from build123d import *

# Parameters (mm, degrees)
BOSS_EXTRUDE1_DEPTH      = 5
SKETCH2_W                = 1
SKETCH2_H                = 2
SKETCH2_W_2              = 2
SKETCH2_H_2              = 30.5
BOSS_EXTRUDE2_DEPTH      = 2
FILLET1_R                = 4
BOSS_EXTRUDE3_DEPTH      = 5
BOSS_EXTRUDE3_DEPTH_BACK = 0.5
SKETCH3_R                = 0.75
FILLET3_R                = 1


with BuildPart() as part:
    # Sketch1 → Boss-Extrude1 (new body)
    with BuildSketch(Plane(origin=(0, 0, 0), x_dir=(1, 0, 0), z_dir=(0, 1, 0))):
        with BuildLine():
            Line((0, 14.4), (25, 14.4))
            ThreePointArc((25, 14.4), (39.4, 0), (25, -14.4))
            Line((25, -14.4), (0, -14.4))
            ThreePointArc((0, -14.4), (-14.4, 0), (0, 14.4))
        make_face()
        with BuildLine():
            Line((0, 12.4), (25, 12.4))
            ThreePointArc((25, 12.4), (37.4, 0), (25, -12.4))
            Line((25, -12.4), (0, -12.4))
            ThreePointArc((0, -12.4), (-12.4, 0), (0, 12.4))
        make_face(mode=Mode.SUBTRACT)
    extrude(amount=BOSS_EXTRUDE1_DEPTH)

    # Sketch2 → Boss-Extrude2 (add)
    with BuildSketch(Plane.XZ):
        with Locations((56.9, 32.5)):
            Rectangle(SKETCH2_W, SKETCH2_H)
        with Locations((55.4, 32.5)):
            Rectangle(SKETCH2_W_2, SKETCH2_H)
        with Locations((55.4, 16.25)):
            Rectangle(SKETCH2_W_2, SKETCH2_H_2)
        with BuildLine():
            Line((39.365235814, -1), (54.4, -1))
            Line((54.4, -1), (54.4, 1))
            Line((54.4, 1), (39.365235814, 1))
            ThreePointArc((39.365235814, 1), (39.4, 0), (39.365235814, -1))
        make_face()
        with Locations((55.4, 0)):
            Rectangle(SKETCH2_W_2, SKETCH2_H)
        with BuildLine():
            Line((37.4, -1), (39.365235814, -1))
            ThreePointArc((39.365235814, -1), (39.4, 0), (39.365235814, 1))
            Line((39.365235814, 1), (37.4, 1))
            Line((37.4, 1), (37.4, -1))
        make_face()
    extrude(amount=-BOSS_EXTRUDE2_DEPTH)

    # Fillet1
    # the kernel refuses this fillet: 4 mm, written as the material it adds along each edge
    with BuildSketch(Plane(origin=(25, 2, 0), x_dir=(0.7371891614816782, 0, -0.6756864214959037), z_dir=(-0.6756864214959037, 0, -0.7371891614816782))) as fillet1_piece_1_section:
        with BuildLine():
            CenterArc((18.272983346, -4), FILLET1_R, 90, 75.522487814)
            Line((18.272983346, 0), (18.272983346, 0.08))
            Line((18.272983346, 0.08), (14.4, 0.08))
            Line((14.4, 0.08), (14.32, 0))
            ThreePointArc((14.32, 0), (14.32, -1.5), (14.322540333, -2.98))
            Line((14.322540333, -2.98), (14.4, -3))
        make_face()
    fillet1_piece_1 = revolve(axis=Axis((25, 2, 0), (0, -1, 0)), revolution_arc=85.014954966, mode=Mode.PRIVATE)
    fillet1_piece_1 = split(fillet1_piece_1, bisect_by=Plane(origin=(40.301586348, 2.758397987, -1), z_dir=(0, 0, 1)), keep=Keep.TOP, mode=Mode.PRIVATE)
    fillet1_piece_1 = split(fillet1_piece_1, bisect_by=Plane(origin=(40.301586348, 2.758397987, 1), z_dir=(0, 0, -1)), keep=Keep.TOP, mode=Mode.PRIVATE)
    add(fillet1_piece_1)
    with BuildSketch(Plane(origin=(39.365235814, 2, 1), x_dir=(-0.17149804582148107, 0, 0.9851844600273663), z_dir=(0, -1, 0))) as fillet1_piece_2:
        with BuildLine():
            CenterArc((3.367524545, -3.978862537), FILLET1_R, 95.892851455, 74.232218513)
            Line((-0.573213295, -3.292870354), (-0.652028052, -3.27915051))
            Line((-0.652028052, -3.27915051), (-0.078814757, 0.013719844))
            Line((-0.078814757, 0.013719844), (0.008213474, 0.079577251))
            ThreePointArc((0.008213474, 0.079577251), (1.47842541, 0.003905135), (2.948637345, 0.079577251))
            Line((2.948637345, 0.079577251), (2.95685082, 0))
        make_face()
    extrude(amount=2)
    with BuildSketch(Plane(origin=(39.365235814, 2, -1), x_dir=(-0.17149804582148342, 0, -0.9851844600273658), z_dir=(0, -1, 0))) as fillet1_piece_3:
        with BuildLine():
            CenterArc((3.367524545, 3.978862537), FILLET1_R, 189.874930032, 74.232218513)
            Line((-0.573213295, 3.292870354), (-0.652028052, 3.27915051))
            Line((-0.652028052, 3.27915051), (-0.078814757, -0.013719844))
            Line((-0.078814757, -0.013719844), (0.008213474, -0.079577251))
            ThreePointArc((0.008213474, -0.079577251), (1.47842541, -0.003905135), (2.948637345, -0.079577251))
            Line((2.948637345, -0.079577251), (2.95685082, 0))
        make_face()
    extrude(amount=2)
    with BuildSketch(Plane(origin=(54.4, 0, 1), x_dir=(-1, 0, 0), z_dir=(0, 1, 0))) as fillet1_piece_4:
        with BuildLine():
            CenterArc((FILLET1_R, FILLET1_R), FILLET1_R, 180, 90)
            Line((0, FILLET1_R), (-FILLET1_R * 0.02, FILLET1_R))
            Line((-FILLET1_R * 0.02, FILLET1_R), (-FILLET1_R * 0.02, -FILLET1_R * 0.02))
            Line((-FILLET1_R * 0.02, -FILLET1_R * 0.02), (FILLET1_R, -FILLET1_R * 0.02))
            Line((FILLET1_R, -FILLET1_R * 0.02), (FILLET1_R, 0))
        make_face()
    extrude(amount=2)
    with BuildSketch(Plane(origin=(56.4, 0, 31.5), x_dir=(0, 0, -1), z_dir=(0, 1, 0))) as fillet1_piece_5:
        with BuildLine():
            CenterArc((2.645751311, -4), FILLET1_R, 90, 41.409622109)
            Line((0, -1), (-0.052915026, -0.94))
            ThreePointArc((-0.052915026, -0.94), (-0.08, -0.5), (-0.08, 0))
            Line((-0.08, 0), (0, 0.08))
            Line((0, 0.08), (2.645751311, 0.08))
            Line((2.645751311, 0.08), (2.645751311, 0))
        make_face()
    extrude(amount=2)
    with BuildSketch(Plane(origin=(39.365235814, 10.355974154, -1), x_dir=(-0.1714980458214834, 0, -0.9851844600273658), z_dir=(0, -1, 0))) as fillet1_piece_6a_section:
        with BuildLine():
            CenterArc((3.367524545, 3.978862537), FILLET1_R, 189.874930032, 74.232218513)
            Line((-0.573213295, 3.292870354), (-0.652028052, 3.27915051))
            Line((-0.652028052, 3.27915051), (-0.078814757, -0.013719844))
            Line((-0.078814757, -0.013719844), (0.008213474, -0.079577251))
            ThreePointArc((0.008213474, -0.079577251), (1.47842541, -0.003905135), (2.948637345, -0.079577251))
            Line((2.948637345, -0.079577251), (2.95685082, 0))
        make_face()
    fillet1_piece_6a = extrude(amount=10.355974154, mode=Mode.PRIVATE)
    fillet1_piece_6a = split(fillet1_piece_6a, bisect_by=Plane(origin=(40.057221624, 5, -1.646357347), z_dir=(0, -1, 0)), keep=Keep.TOP, mode=Mode.PRIVATE)
    fillet1_piece_6a = split(fillet1_piece_6a, bisect_by=Plane(origin=(40.057221624, 2, -1.646357347), z_dir=(0, 1, 0)), keep=Keep.TOP, mode=Mode.PRIVATE)
    with BuildSketch(Plane(origin=(25, 2, 0), x_dir=(0.7371891614816782, 0, -0.6756864214959037), z_dir=(-0.6756864214959037, 0, -0.7371891614816782))) as fillet1_piece_6b_section:
        with BuildLine():
            CenterArc((18.272983346, -4), FILLET1_R, 90, 75.522487814)
            Line((18.272983346, 0), (18.272983346, 0.08))
            Line((18.272983346, 0.08), (14.4, 0.08))
            Line((14.4, 0.08), (14.32, 0))
            ThreePointArc((14.32, 0), (14.32, -1.5), (14.322540333, -2.98))
            Line((14.322540333, -2.98), (14.4, -3))
        make_face()
    fillet1_piece_6b = revolve(axis=Axis((25, 2, 0), (0, -1, 0)), revolution_arc=85.014954966, mode=Mode.PRIVATE)
    fillet1_piece_6b = split(fillet1_piece_6b, bisect_by=Plane(origin=(38.861424428, 2.733448244, -1), z_dir=(0, 0, -1)), keep=Keep.TOP, mode=Mode.PRIVATE)
    fillet1_piece_6 = fillet1_piece_6a & fillet1_piece_6b
    add(fillet1_piece_6)
    with BuildSketch(Plane(origin=(25, 2, 0), x_dir=(0.7371891614816782, 0, -0.6756864214959037), z_dir=(-0.6756864214959037, 0, -0.7371891614816782))) as fillet1_piece_7a_section:
        with BuildLine():
            CenterArc((18.272983346, -4), FILLET1_R, 90, 75.522487814)
            Line((18.272983346, 0), (18.272983346, 0.08))
            Line((18.272983346, 0.08), (14.4, 0.08))
            Line((14.4, 0.08), (14.32, 0))
            ThreePointArc((14.32, 0), (14.32, -1.5), (14.322540333, -2.98))
            Line((14.322540333, -2.98), (14.4, -3))
        make_face()
    fillet1_piece_7a = revolve(axis=Axis((25, 2, 0), (0, -1, 0)), revolution_arc=85.014954966, mode=Mode.PRIVATE)
    fillet1_piece_7a = split(fillet1_piece_7a, bisect_by=Plane(origin=(38.861423807, 2.733448455, 1), z_dir=(0, 0, 1)), keep=Keep.TOP, mode=Mode.PRIVATE)
    with BuildSketch(Plane(origin=(39.365235814, 10.355974154, 1), x_dir=(-0.17149804582148107, 0, 0.9851844600273663), z_dir=(0, -1, 0))) as fillet1_piece_7b_section:
        with BuildLine():
            CenterArc((3.367524545, -3.978862537), FILLET1_R, 95.892851455, 74.232218513)
            Line((-0.573213295, -3.292870354), (-0.652028052, -3.27915051))
            Line((-0.652028052, -3.27915051), (-0.078814757, 0.013719844))
            Line((-0.078814757, 0.013719844), (0.008213474, 0.079577251))
            ThreePointArc((0.008213474, 0.079577251), (1.47842541, 0.003905135), (2.948637345, 0.079577251))
            Line((2.948637345, 0.079577251), (2.95685082, 0))
        make_face()
    fillet1_piece_7b = extrude(amount=10.355974154, mode=Mode.PRIVATE)
    fillet1_piece_7b = split(fillet1_piece_7b, bisect_by=Plane(origin=(40.057221624, 5, 1.646357347), z_dir=(0, -1, 0)), keep=Keep.TOP, mode=Mode.PRIVATE)
    fillet1_piece_7b = split(fillet1_piece_7b, bisect_by=Plane(origin=(40.057221624, 2, 1.646357347), z_dir=(0, 1, 0)), keep=Keep.TOP, mode=Mode.PRIVATE)
    fillet1_piece_7 = fillet1_piece_7a & fillet1_piece_7b
    add(fillet1_piece_7)
    # the kernel refuses this fillet: 4 mm, written as the material it takes off along each edge
    with BuildSketch(Plane(origin=(56.4, -10, -1), x_dir=(-1, 0, 0), z_dir=(0, 1, 0))) as fillet1_2_piece_1:
        with BuildLine():
            CenterArc((FILLET1_R, FILLET1_R), FILLET1_R, 180, 90)
            Line((0, FILLET1_R), (-FILLET1_R * 0.02, FILLET1_R))
            Line((-FILLET1_R * 0.02, FILLET1_R), (-FILLET1_R * 0.02, -FILLET1_R * 0.02))
            Line((-FILLET1_R * 0.02, -FILLET1_R * 0.02), (FILLET1_R, -FILLET1_R * 0.02))
            Line((FILLET1_R, -FILLET1_R * 0.02), (FILLET1_R, 0))
        make_face()
    extrude(amount=22, mode=Mode.SUBTRACT)
    with BuildSketch(Plane(origin=(54.4, -9.682458366, 33.5), x_dir=(1, 0, 0), z_dir=(0, 1, 0))) as fillet1_2_piece_2:
        with BuildLine():
            CenterArc((4, 3.872983346), FILLET1_R, 180, 75.522487814)
            Line((0, 3.872983346), (-0.08, 3.872983346))
            Line((-0.08, 3.872983346), (-0.08, 0))
            Line((-0.08, 0), (0, -0.08))
            ThreePointArc((0, -0.08), (1.5, -0.08), (2.98, -0.077459667))
            Line((2.98, -0.077459667), (3, 0))
        make_face()
    extrude(amount=21.364916731, mode=Mode.SUBTRACT)

    # Sketch3 → Boss-Extrude3 (add, two sides: drawn at the far end of the back side and taken through both)
    with BuildSketch(Plane(origin=(57.4, 0, 0), x_dir=(0, 0, -1), z_dir=(1, 0, 0)).offset(-BOSS_EXTRUDE3_DEPTH_BACK)):
        with Locations((-32.5, 0)):
            Circle(SKETCH3_R)
    extrude(amount=BOSS_EXTRUDE3_DEPTH + BOSS_EXTRUDE3_DEPTH_BACK)

    # Fillet3
    # the kernel refuses this fillet: 1 mm, written as the material it adds along each edge
    with BuildSketch(Plane(origin=(57.4, 0, 32.5), x_dir=(0, 0, -1), z_dir=(0, -1, 0))) as fillet3_piece_1_section:
        with BuildLine():
            CenterArc((0.75 + FILLET3_R, FILLET3_R), FILLET3_R, 180, 90)
            Line((0.75, FILLET3_R), (0.75, 0))
            Line((0.75, 0), (0.75 + FILLET3_R, 0))
        make_face()
    fillet3_piece_1 = revolve(axis=Axis((57.4, 0, 32.5), (1, 0, 0)), revolution_arc=180, mode=Mode.PRIVATE)
    fillet3_piece_1 = fillet3_piece_1 & Plane(origin=(58.4, 0.745327828, 29.627016654), x_dir=(1, 0, 0), z_dir=(0, -1, 0)) * Cylinder(4, 7, mode=Mode.PRIVATE)
    fillet3_piece_1 = fillet3_piece_1 - Plane(origin=(60.4, 0.745327828, 28.854248689), x_dir=(0, 0, -1), z_dir=(0, -1, 0)) * Cylinder(4, 7, mode=Mode.PRIVATE)
    add(fillet3_piece_1)


solid = part.part
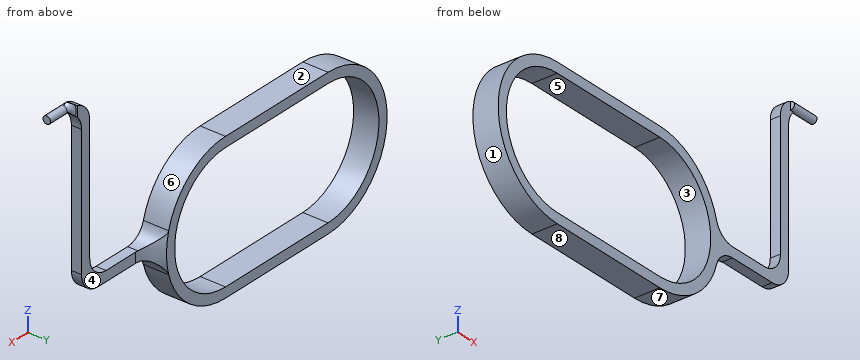
Work out the finished part from the listing and answer in its coordinate system (mm). Face numbers are marked on the shaded views. A direction names the side the tool comes from. Round coordinates to 2 decimals unless told otherwise and drop trailing zeros. Write each loop counter-clockwise with the first axis right and the second up, starting at its lowest first coordinate (ties: lowest second). Pieces come first, ordered by that corner, then holes. Notation, with made-up numbers: (-30.75, 41.5) - (3.25, 41.5) arc R35 ccw to (3.25, 79.5) - close; hole circle Ø7 at (30, 45.5). An arc over 180 degrees is marked (long way). Answer in a Markdown table with one row per item. Add a question column.
1. A cutting plane is placed at D-D, the plane x = 35. Determine the outline of the cut face in (y, z).
2. A cutting plane is placed at B-B, the plane z = 0. Determine the outline of the cut face in (x, y).
3. A cutting plane is placed at C-C, the plane z = 18.5. Determine the outline of the cut face in (x, y).
4. Find the intervals of material crossed by line 1 along X through (y, z) = (1.95, 3.5); line 2 along Z through (x, y) = (-0.5, 2.65); line 3 along X through (y, z) = (0.45, 29), in increasing order. Write a range as from..to.
5. A cutting plane is placed at A-A, the plane x = 3. Determine the outline of the cut face in (y, z), and give its area (3 significant figures).
6. The mould has two halves that part along X. Classify the marked faces 1, 2 and 3: +X half, -X half, draft (parallel to the pull), parting line (faces both ways), or undercut.
7. For the marked faces 4, 5, 6, 7 and 8, determine the directions among +Z, -Z, +X, -X, +Y, -Y from which every point of the face is accessible in a straight line to the end or side of a thin tool.
8. Given pin 1 (0.6 mm diameter, centred on y = 1, z = 18, fed in from +X); pin 2 (1 mm diameter, centred on x = 49.5, y = 1.5, fed in from -Z); pin 3 (2 mm diameter, centred on x = 22, y = 4, fed in from +Z); pin 4 (12 mm diameter, centred on x = 8, z = 2.5, fed in from -Y), each flat-ended and moving along its own axis, determine where each tip first touches the part or whether it passes through.
Worked out:
| question | item | result |
|---|---|---|
| 1 | outline | (0, -10.36) - (5, -10.36) - (5, -7.33) - (0, -7.33) - close; (0, 7.33) - (5, 7.33) - (5, 10.36) - (0, 10.36) - close |
| 2 | outline | (-14.4, 0) - (-12.4, 0) - (-12.4, 5) - (-14.4, 5) - close; (37.4, 0) - (55.05, 0) - (55.05, 2) - (43.27, 2) arc R4 cw to (39.4, 5) - (37.4, 5) - close |
| 3 | outline | (54.4, 0) - (56.4, 0) - (56.4, 2) - (54.4, 2) - close |
| 4 | line 1 | -13.97..-11.9, 36.9..39, 54.11..56.4 |
| 4 | line 2 | -14.39..-12.39, 12.39..14.39 |
| 4 | line 3 | 54.4..56.4 |
| 5 | outline | (0, -14.4) - (5, -14.4) - (5, -12.4) - (0, -12.4) - close; (0, 12.4) - (5, 12.4) - (5, 14.4) - (0, 14.4) - close |
| 5 | area | 20.0 mm^2 |
| 6 | face 1 | -X half |
| 6 | face 2 | draft |
| 6 | face 3 | undercut |
| 7 | face 4 | +Z, -Z, +X, +Y |
| 7 | face 5 | +Y, -Y |
| 7 | face 6 | +Z, +Y, -Y |
| 7 | face 7 | -Z, +X, +Y, -Y |
| 7 | face 8 | -Z, +X, -X, +Y, -Y |
| 8 | pin 1 | x = 56.4 |
| 8 | pin 2 | z = -1 |
| 8 | pin 3 | z = 14.4 |
| 8 | pin 4 | through |
